```python
from build123d import *

# Parameters (mm, degrees)
SKETCH1_W           = 127
SKETCH1_H           = 228.6
SKETCH1_R           = 3.175
BOSS_EXTRUDE1_DEPTH = 6.35


with BuildPart() as part:
    # Sketch1 → Boss-Extrude1 (new body)
    with BuildSketch(Plane(origin=(0, 0, 0), x_dir=(1, 0, 0), z_dir=(0, 1, 0))):
        Rectangle(SKETCH1_W, SKETCH1_H)
        with Locations(Location((-57.15, 107.95, 0), (0, 0, 270))):
            Circle(SKETCH1_R, mode=Mode.SUBTRACT)
        with Locations(Location((-57.15, 69.85, 0), (0, 0, 270))):
            Circle(SKETCH1_R, mode=Mode.SUBTRACT)
        with Locations(Location((-31.75, 107.95, 0), (0, 0, 270))):
            Circle(SKETCH1_R, mode=Mode.SUBTRACT)
        with Locations(Location((-31.75, 69.85, 0), (0, 0, 270))):
            Circle(SKETCH1_R, mode=Mode.SUBTRACT)
        with Locations(Location((-31.75, -69.85, 0), (0, 0, 90))):
            Circle(SKETCH1_R, mode=Mode.SUBTRACT)
        with Locations(Location((-57.15, -69.85, 0), (0, 0, 90))):
            Circle(SKETCH1_R, mode=Mode.SUBTRACT)
        with Locations(Location((-31.75, -107.95, 0), (0, 0, 90))):
            Circle(SKETCH1_R, mode=Mode.SUBTRACT)
        with Locations(Location((-57.15, -107.95, 0), (0, 0, 90))):
            Circle(SKETCH1_R, mode=Mode.SUBTRACT)
        with Locations(Location((57.15, 98.425, 0), (0, 0, 270))):
            Circle(SKETCH1_R, mode=Mode.SUBTRACT)
        with Locations(Location((31.75, 98.425, 0), (0, 0, 270))):
            Circle(SKETCH1_R, mode=Mode.SUBTRACT)
        with Locations(Location((57.15, 79.375, 0), (0, 0, 270))):
            Circle(SKETCH1_R, mode=Mode.SUBTRACT)
        with Locations(Location((31.75, 79.375, 0), (0, 0, 270))):
            Circle(SKETCH1_R, mode=Mode.SUBTRACT)
        with Locations(Location((57.15, -88.9, 0), (0, 0, 270))):
            Circle(SKETCH1_R, mode=Mode.SUBTRACT)
        with Locations(Location((19.05, -88.9, 0), (0, 0, 270))):
            Circle(SKETCH1_R, mode=Mode.SUBTRACT)
        with Locations(Location((-53.848, -53.975, 0), (0, 0, 270))):
            Circle(SKETCH1_R, mode=Mode.SUBTRACT)
        with Locations(Location((-53.848, 53.975, 0), (0, 0, 90))):
            Circle(SKETCH1_R, mode=Mode.SUBTRACT)
        with Locations(Location((53.848, -53.975, 0), (0, 0, 90))):
            Circle(SKETCH1_R, mode=Mode.SUBTRACT)
        with Locations(Location((53.848, 53.975, 0), (0, 0, 270))):
            Circle(SKETCH1_R, mode=Mode.SUBTRACT)
        with Locations(Location((-3.175, -82.55, 0), (0, 0, 270))):
            Circle(SKETCH1_R, mode=Mode.SUBTRACT)
        with Locations(Location((-3.175, -95.25, 0), (0, 0, 270))):
            Circle(SKETCH1_R, mode=Mode.SUBTRACT)
        Polygon((-53.975, -101.599988436), (-53.940723216, -76.200011564), (-28.575, -76.200011564), (-28.575, -101.599988436), align=None, mode=Mode.SUBTRACT)
        Polygon((-53.975, 101.599988436), (-53.940723216, 76.200011564), (-28.575, 76.200011564), (-28.575, 101.599988436), align=None, mode=Mode.SUBTRACT)
    extrude(amount=BOSS_EXTRUDE1_DEPTH)


solid = part.part
```
Check sheet for the modelled part. Datum: model origin and axes. Units: mm. A direction names the side the tool comes from. Coordinates: 2 decimals unless noted, no trailing zeros. Order: outer loops, then holes, each group sorted by start corner. A loop starts at its lowest first (then second) coordinate and runs counter-clockwise, first axis right, second up. Notation, with made-up numbers: (47, 39) -> (78, 39) arc R21 cw to (78, 63) -> close; hole circle Ø9 at (68, 57.5). An arc over 180 degrees is marked (long way). Write item = value, one per line. Start each with the question number.
1) Access from +Z, -Z, +X, -X, +Y, -Y to the whole of each face (thin tool, end or side, straight path). Record for faces 5 (the flat face through (-28.575, 3, 89)), 6 (the flat face through (-1, 3, -114.3)).
2) Material ranges on L1, parallel to X at y = 4.75, z = 107.95 (3 decimals); L2, parallel to Z at x = -50, y = 5.25; L3, parallel to X at y = 3.5, z = -79.5 (3 decimals), recorded low to high.
3) Mould release check, pull along X, two halves, no side actions. Record for faces 1 (the cylindrical face through (-50.749, 3.131, -53.287)), 2 (the flat face through (-41, 3, 101.6)), 3 (the flat face through (-63.5, 3, 2)), 4 (the flat face through (-1, 3, 114.3)): +X half, -X half, draft (parallel to the pull), parting line (faces both ways), or undercut.
4) Cross-section at A-A (x = 31.75). Enter the section's corners in (y, z).
5) Go/stop test with a flat-tipped pin: P1, Ø5, axis at x = -31.75, z = -69.85, coming from the +Y side. Record where the tip stops, or that it passes through.
6) Cross-section at B-B (z = 107.95). Enter the section's corners in (x, y) (3 decimals), then the cut area to 3 significant figures.
7) Cross-section at C-C (x = -31.75). Enter the section's corners in (y, z) (3 decimals), then the cut area to 3 significant figures.
8) Cross-section at D-D (z = -88). Enter the section's corners in (x, y) (3 decimals).
Ans:
q1.face_5 = +Y, -Y
q1.face_6 = -Z, +X, -X, +Y, -Y
q2.L1 = -63.5 to -60.325, -53.975 to -34.925, -28.575 to 63.5
q2.L2 = -114.3 to -101.6, -76.2 to 76.2, 101.6 to 114.3
q2.L3 = -63.5 to -53.945, -28.575 to 28.577, 34.923 to 53.977, 60.323 to 63.5
q3.face_1 = undercut
q3.face_2 = undercut
q3.face_3 = -X half
q3.face_4 = draft
q4.outline = (0, -114.3) -> (6.35, -114.3) -> (6.35, -101.6) -> (0, -101.6) -> close; (0, -95.25) -> (6.35, -95.25) -> (6.35, -82.55) -> (0, -82.55) -> close; (0, -76.2) -> (6.35, -76.2) -> (6.35, 114.3) -> (0, 114.3) -> close
q5.P1 = through
q6.outline = (-63.5, 0) -> (-60.325, 0) -> (-60.325, 6.35) -> (-63.5, 6.35) -> close; (-53.975, 0) -> (-34.925, 0) -> (-34.925, 6.35) -> (-53.975, 6.35) -> close; (-28.575, 0) -> (63.5, 0) -> (63.5, 6.35) -> (-28.575, 6.35) -> close
q6.area = 726 mm²
q7.outline = (0, -114.3) -> (6.35, -114.3) -> (6.35, -111.125) -> (0, -111.125) -> close; (0, -104.775) -> (6.35, -104.775) -> (6.35, -101.6) -> (0, -101.6) -> close; (0, -76.2) -> (6.35, -76.2) -> (6.35, -73.025) -> (0, -73.025) -> close; (0, -66.675) -> (6.35, -66.675) -> (6.35, 66.675) -> (0, 66.675) -> close; (0, 73.025) -> (6.35, 73.025) -> (6.35, 76.2) -> (0, 76.2) -> close; (0, 101.6) -> (6.35, 101.6) -> (6.35, 104.775) -> (0, 104.775) -> close; (0, 111.125) -> (6.35, 111.125) -> (6.35, 114.3) -> (0, 114.3) -> close
q7.area = 968 mm²
q8.outline = (-63.5, 0) -> (-53.957, 0) -> (-53.957, 6.35) -> (-63.5, 6.35) -> close; (-28.575, 0) -> (63.5, 0) -> (63.5, 6.35) -> (-28.575, 6.35) -> close
